Model file for the job. Use its own axes, mm. A direction names the side the tool comes from. Coordinates: 2 decimals unless noted, no trailing zeros. Order: outer loops, then holes, each group sorted by start corner. A loop starts at its lowest first (then second) coordinate and runs counter-clockwise, first axis right, second up. Notation, with made-up numbers: (33, -9) -> (63, -9) arc R29 ccw to (63, 21) -> close; hole circle Ø1 at (33, 12). An arc over 180 degrees is marked (long way). Return JSON: item names as keys, results as strings. Group by question number.
1) Flat gauge pins, fed straight in: pin 1 (8 mm diameter, centred on x = 12.5, y = -11, fed in from -Z); pin 2 (5 mm diameter, centred on x = -1, z = -2, fed in from -Y); pin 3 (10 mm diameter, centred on x = 2.5, y = -16.5, fed in from +Z); pin 4 (4 mm diameter, centred on x = 13, y = -0.5, fed in from +Z). Where does each tip first touch, or does it go through?
2) Pull direction Y, two halves, no side cores. Call faces 1 (the flat face through (15.723, 9.5, 0.3)), 2 (the cylindrical face through (3.36, -14.18, -1.86)), 3 (the cylindrical face through (14.202, 21.477, -4.769)): +Y half, -Y half, draft (parallel to the pull), parting line (faces both ways), or undercut.
3) Probe line 1 (Y direction, x = 13.4, z = 0); line 2 (X direction, y = 1, z = 11); line 3 (Z direction, x = 2.5, y = 0). List the from-to ranges inside material, lowest first.
4) Cut at C-C (x = 4.5). Write the cut outline in (y, z), and give its area (3 significant figures).
5) Cut at A-A (z = 0). Write the cut outline in (x, y).
6) Which spindle directions (+Z, -Z, +X, -X, +Y, -Y) get a long thin tool onto all of the face, cutting with end or side? Do faces 4 (the flat face through (12.723, 9, 3)), 5 (the cylindrical face through (14.24, -7.84, 5)). Say none if no direction does.
7) Cut at D-D (x = 7.25). Write the cut outline in (y, z).
from build123d import *


with BuildPart() as f1:
    # F0 (on Front) → F1 (revolve)
    with BuildSketch(Plane.XZ):
        with BuildLine():
            Line((-6.277208, 22), (-6.277208, 14.3))
            Line((-6.277208, 14.3), (12.722792, 14.3))
            Line((12.722792, 14.3), (12.722792, 9.3))
            Line((12.722792, 9.3), (15.722792, 9.3))
            Line((15.722792, 9.3), (15.722792, 22))
            Line((15.722792, 22), (12.722792, 22))
            ThreePointArc((12.722792, 22), (4.722792, 18), (-3.277208, 22))
            Line((-3.277208, 22), (-6.277208, 22))
        make_face()
    revolve(axis=Axis((-0.613183, 0, 0), (1, 0, 0)))


solid = f1.part
Answers below:
{
 "1": {"pin 1": "stops at z = -20.85", "pin 2": "stops at y = -21.98", "pin 3": "stops at z = 15", "pin 4": "stops at z = 22"},
 "2": {"face 1": "draft", "face 2": "undercut", "face 3": "parting line"},
 "3": {"line 1": "y = -22 to -9.3, 9.3 to 22", "line 2": "x = 12.72 to 15.72", "line 3": "z = -18.25 to -14.3, 14.3 to 18.25"},
 "4": {"outline": "circle Ø36 at (0, 0); hole circle Ø28.6 at (0, 0)", "area": "376 mm^2"},
 "5": {"outline": "(-6.28, -22) -> (-3.28, -22) arc R10 cw to (12.72, -22) -> (15.72, -22) -> (15.72, -9.3) -> (12.72, -9.3) -> (12.72, -14.3) -> (-6.28, -14.3) -> close; (-6.28, 14.3) -> (12.72, 14.3) -> (12.72, 9.3) -> (15.72, 9.3) -> (15.72, 22) -> (12.72, 22) arc R10 cw to (-3.28, 22) -> (-6.28, 22) -> close"},
 "6": {"face 4": "-X", "face 5": "+X, -X"},
 "7": {"outline": "circle Ø36.65 at (0, 0); hole circle Ø28.6 at (0, 0)"}
}
